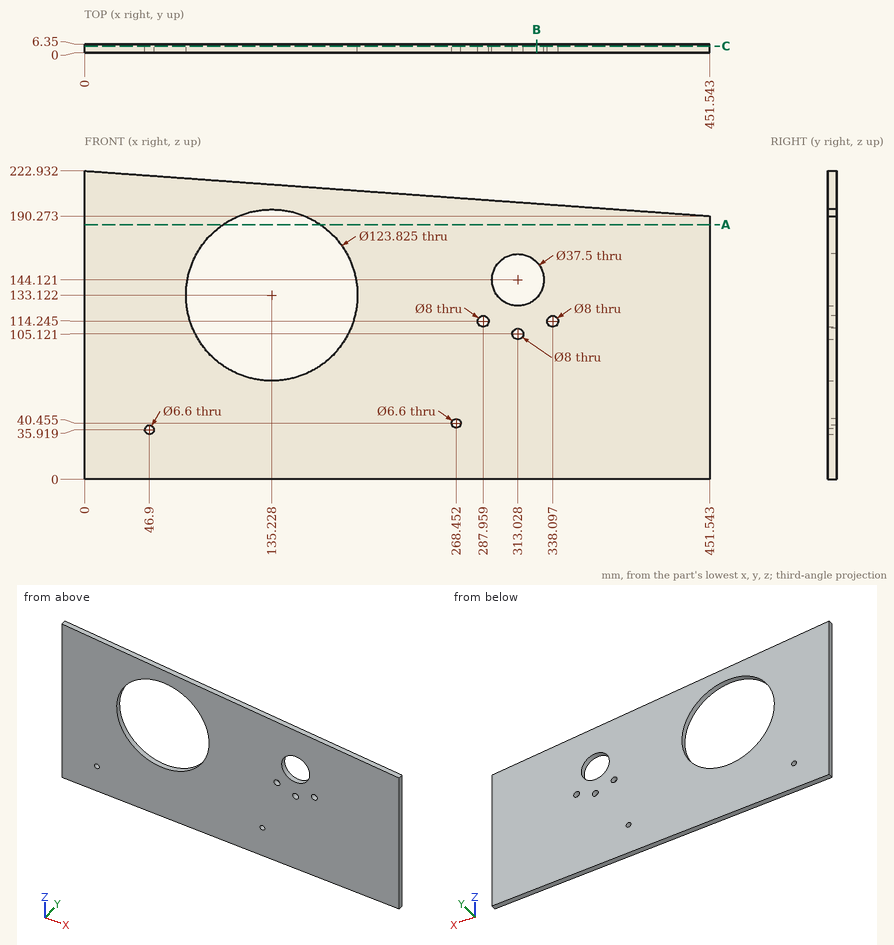
Verification items for this drawing (mm, ordinates from the low corner). Coordinates: 2 decimals unless noted, no trailing zeros. Loops run counter-clockwise (first coordinate to the right, second up) from the corner with the lowest first, then second, coordinate; pieces in that order, holes last. Notation, with made-up numbers: (58.5, 11.25) - (98.5, 11.25) arc R10 cw to (98.5, 23.25) - close; hole circle Ø8 at (49, -9.5). An arc over 180 degrees is marked (long way). Answer as a JSON object with one key per item and string values.
(1) Scan lines: line 1 along Z through (x, y) = (290, 4) (1 decimal); line 2 along X through (y, z) = (5.5, 88.5) (1 decimal); line 3 along X through (y, z) = (1.75, 42) (1 decimal). Record each from-to range of solid material in increasing order.
Response:
{"line 1": "z = 0 to 110.8, 117.7 to 202", "line 2": "x = 0 to 92.3, 178.1 to 451.5", "line 3": "x = 0 to 265.5, 271.4 to 451.5"}
(2) Cross-section at B-B, the plane x = 326.5. Record the boundary of the cut face in (y, z), then the cut area to 3 significant figures.
Response:
{"outline": "(0, 0) - (6.35, 0) - (6.35, 131.08) - (0, 131.08) - close; (0, 157.16) - (6.35, 157.16) - (6.35, 199.32) - (0, 199.32) - close", "area": "1,100 mm²"}
(3) Cross-section at A-A, the plane z = 184. Record the boundary of the cut face in (x, y).
Response:
{"outline": "(0, 0) - (99.95, 0) - (99.95, 6.35) - (0, 6.35) - close; (170.51, 0) - (451.54, 0) - (451.54, 6.35) - (170.51, 6.35) - close"}
(4) Cross-section at C-C, the plane y = 4.75. Count the separate pieces of the cut face and the enclosed holes in it, then the cut area to 3 significant figures.
Response:
{"separate pieces": "1", "enclosed holes": "7", "area": "79,900 mm²"}
(5) Go/stop test with a flat-tipped pin: pin 1 Ø10.5 at (x, z) = (268.45, 40.45) entering from +Y. Record where the tip stops, or that it passes through.
Response:
{"pin 1": "stops at y = 6.35"}
